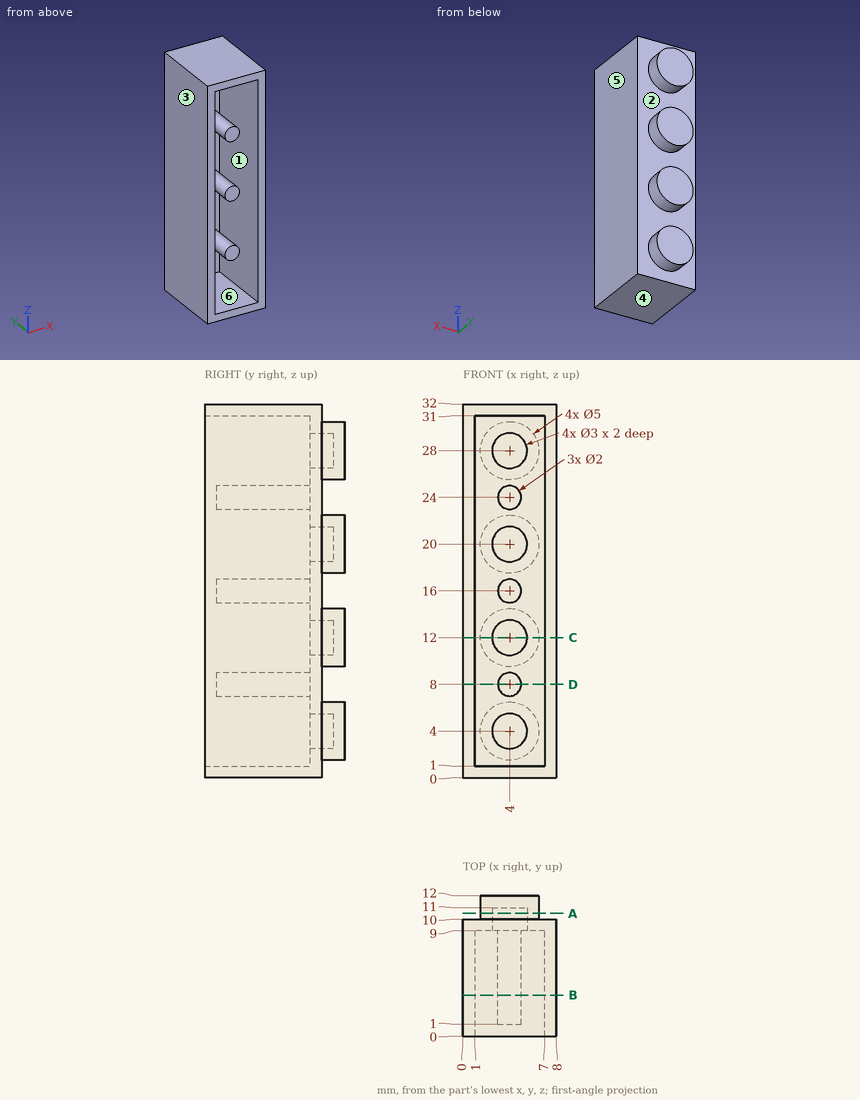
Part print with two shaded views. Sizes in mm from the minimum x, y, z corner. A direction names the side the tool comes from. Give positions to 0.01 mm unless a question says otherwise; leave off trailing zeros. Loops run counter-clockwise (first coordinate to the right, second up) from the corner with the lowest first, then second, coordinate; pieces in that order, holes last. Notation, with made-up numbers: (-1.5, 30.5) - (38.5, 30.5) arc R21 cw to (38.5, 53.5) - close; hole circle Ø2 at (86.25, 77). An arc over 180 degrees is marked (long way). Put each result on its own line as item: value.
Q1. Probe line 1 along Z through (x, y) = (4, 9.95); line 2 along Z through (x, y) = (4, 1.75); line 3 along X through (y, z) = (9.8, 12). List the from-to ranges inside material, lowest first.
Filled in:
line 1: z = 0 to 2.5, 5.5 to 10.5, 13.5 to 18.5, 21.5 to 26.5, 29.5 to 32
line 2: z = 0 to 1, 7 to 9, 15 to 17, 23 to 25, 31 to 32
line 3: x = 0 to 2.5, 5.5 to 8
Q2. Slice it at C-C (z = 12). Give the cut face in (x, y), plus the area to 3 significant figures.
Filled in:
outline: (0, 0) - (1, 0) - (1, 9) - (2.5, 9) - (2.5, 11) - (5.5, 11) - (5.5, 9) - (7, 9) - (7, 0) - (8, 0) - (8, 10) - (6.5, 10) - (6.5, 12) - (1.5, 12) - (1.5, 10) - (0, 10) - close
area: 30.0 mm²
Q3. Slice it at D-D (z = 8). Give the cut face in (x, y), plus the area to 3 significant figures.
Filled in:
outline: (0, 0) - (1, 0) - (1, 9) - (3, 9) - (3, 1) - (5, 1) - (5, 9) - (7, 9) - (7, 0) - (8, 0) - (8, 10) - (0, 10) - close
area: 42.0 mm²
Q4. Mould opens along X. For the marked faces 4, 5 and 6 say: pulls with the +X half, pulls with the -X half, needs draft (parallel to the pull), parting line crosses it, or undercut.
Filled in:
face 4: needs draft
face 5: pulls with the +X half
face 6: undercut
Q5. Slice it at A-A (y = 10.5). Give the cut face in (x, z).
Filled in:
outline: circle Ø5 at (4, 4); circle Ø5 at (4, 12); circle Ø5 at (4, 20); circle Ø5 at (4, 28); hole circle Ø3 at (4, 4); hole circle Ø3 at (4, 12); hole circle Ø3 at (4, 20); hole circle Ø3 at (4, 28)
Q6. Slice it at B-B (y = 3.5). Give the cut face in (x, z).
Filled in:
outline: (0, 0) - (8, 0) - (8, 32) - (0, 32) - close; circle Ø2 at (4, 8); circle Ø2 at (4, 16); circle Ø2 at (4, 24); hole (1, 1) - (7, 1) - (7, 31) - (1, 31) - close
Q7. Tool access for the marked faces 1, 2 and 3: list every direction of +Z, -Z, +X, -X, +Y, -Y with a clear straight run to the whole face (end or side of a thin tool).
Filled in:
face 1: -Y
face 2: +Y
face 3: +Z, -Z, -X, +Y, -Y
Q8. Flat gauge pins, fed straight in: pin 1 (2.5 mm diameter, centred on x = 4.5, z = 3.5, fed in from -Y); pin 2 (2 mm diameter, centred on x = 4, z = 16, fed in from -Y); pin 3 (0.9 mm diameter, centred on x = 3.5, z = 28.5, fed in from -Y). Where does each tip first touch, or does it go through?
Filled in:
pin 1: stops at y = 9
pin 2: stops at y = 1
pin 3: stops at y = 11
